from build123d import *

# Parameters (mm, degrees)
BASE_FLANGE2_DEPTH              = 2
M6X1_0_TAPPED_HOLE1_D           = 5
M6X1_0_TAPPED_HOLE1_DEPTH       = 15
M6X1_0_TAPPED_HOLE1_CSINK_D     = 6.05
M6X1_0_TAPPED_HOLE1_CSINK_ANGLE = 90
M6X1_0_TAPPED_HOLE1_TIP         = 1.502151548


# Sheet-metal steps are written as plain solids
with BuildPart() as part:
    # Sketch1 → Base-Flange2 (new body)
    with BuildSketch(Plane.XY):
        Polygon((18.875, 0), (18.875, 82.18171901), (76.986250802, 140.292969812), (50.292969812, 166.986250802), (-18.875, 97.81828099), (-18.875, 0), align=None)
    extrude(amount=-BASE_FLANGE2_DEPTH)

    # M6x1.0 Tapped Hole1
    with Locations(Plane.XY):
        with Locations((42.426406871, 132.426406871), (21.213203436, 111.213203436), (0, 60), (0, 30)):
            CounterSinkHole(M6X1_0_TAPPED_HOLE1_D / 2, M6X1_0_TAPPED_HOLE1_CSINK_D / 2, depth=M6X1_0_TAPPED_HOLE1_DEPTH, counter_sink_angle=M6X1_0_TAPPED_HOLE1_CSINK_ANGLE)
            with Locations((0, 0, -(M6X1_0_TAPPED_HOLE1_DEPTH + M6X1_0_TAPPED_HOLE1_TIP / 2))):  # 118° drill point
                Cone(0, M6X1_0_TAPPED_HOLE1_D / 2, M6X1_0_TAPPED_HOLE1_TIP, mode=Mode.SUBTRACT)


solid = part.part
Could you check a few things on this model? Use its own coordinates, in mm. Round coordinates to 2 decimals unless told otherwise and drop trailing zeros. Order: outer loops, then holes, each group sorted by start corner. A loop starts at its lowest first (then second) coordinate and runs counter-clockwise, first axis right, second up.
Q1. Imagine slicing it at B-B, the plane x = 0. List the corners of the cut face in (y, z) for me (3 decimals), then the cut area to 3 significant figures.
Geometry says:
outline: (0, -2) - (27.5, -2) - (27.5, -0.525) - (26.975, 0) - (0, 0) - close; (32.5, -2) - (57.5, -2) - (57.5, -0.525) - (56.975, 0) - (33.025, 0) - (32.5, -0.525) - close; (62.5, -2) - (116.693, -2) - (116.693, 0) - (63.025, 0) - (62.5, -0.525) - close
area: 213 mm2
Q2. Imagine slicing it at A-A, the plane y = 30. List the corners of the cut face in (x, z) for me (3 decimals), then the cut area to 3 significant figures.
Geometry says:
outline: (-18.875, -2) - (-2.5, -2) - (-2.5, -0.525) - (-3.025, 0) - (-18.875, 0) - close; (2.5, -2) - (18.875, -2) - (18.875, 0) - (3.025, 0) - (2.5, -0.525) - close
area: 65.2 mm2
Q3. Thinking about a two-plate mould opening in X: for faces 1 (the face through (63.83, 153.45, -0.99)), 2 (the face through (0.54, 57.56, -1.27)), 3 (the face through (18, 85, 0)), 4 (the face through (-1.34, 32.11, -1.27)), which applies, released by +X, released by -X, zero draft, split by the parting line, or undercut?
Geometry says:
face 1: released by +X
face 2: undercut
face 3: zero draft
face 4: undercut
Q4. Imagine slicing it at C-C, the plane z = -0.9. List the corners of the cut face in (x, y) for me (3 decimals).
Geometry says:
outline: (-18.875, 0) - (18.875, 0) - (18.875, 82.182) - (76.986, 140.293) - (50.293, 166.986) - (-18.875, 97.818) - close; hole circle Ø5 at (0, 30); hole circle Ø5 at (0, 60); hole circle Ø5 at (21.213, 111.213); hole circle Ø5 at (42.426, 132.426)
Q5. Imagine slicing it at D-D, the plane x = -11. List the corners of the cut face in (y, z) for me.
Geometry says:
outline: (0, -2) - (105.69, -2) - (105.69, 0) - (0, 0) - close
Q6. Please list where these lines run through material, in increasing order: probe 1 along Y at (x, z) = (0, -1.2); probe 2 along X at (y, z) = (134, -1.9); probe 3 along X at (y, z) = (112.5, -0.6).
Geometry says:
probe 1: y = 0 to 27.5, 32.5 to 57.5, 62.5 to 116.69
probe 2: x = 17.31 to 40.48, 44.37 to 70.69
probe 3: x = -4.19 to 19.07, 23.36 to 49.19
Q7. I'm going to push flat-ended pins straight in: P1, Ø8, axis at x = 21.21, y = 111.21, coming from the -Z side; P2, Ø4.5, axis at x = 0, y = 30, coming from the -Z side. Where does each tip first touch, or does it pass through?
Geometry says:
P1: stops at z = -2
P2: passes through
